from build123d import *

# Parameters (mm, degrees)
EXTRUDE_1_DEPTH = 6
FILLET_1_R      = 3
CHAMFER_1_SIZE  = 3


with BuildPart() as part:
    # 草图1 → 凸台-拉伸1 (new body)
    with BuildSketch(Plane.XY):
        Polygon((-25, 0), (25, 0), (25, 10), (9, 10), (9, 19), (-9, 19), (-9, 10), (-25, 10), align=None)
    extrude(amount=EXTRUDE_1_DEPTH)

    # 圆角1
    fillet_1_edges = [part.edges().sort_by_distance(p)[0] for p in [
        (25, 10, 3),
        (25, 0, 3),
        (-25, 0, 3),
        (-25, 10, 3),
    ]]
    fillet(fillet_1_edges, radius=FILLET_1_R)

    # 倒角1
    chamfer_1_edges = [part.edges().sort_by_distance(p)[0] for p in [
        (0, 19, 6),
        (0, 19, 0),
    ]]
    chamfer(chamfer_1_edges, length=CHAMFER_1_SIZE - 0.0001)  # a hair under: the kernel refuses the full size


solid = part.part
The model under review builds one solid part; all positions refer to its coordinate system, in mm. A direction names the side the tool comes from. Coordinates: 2 decimals unless noted, no trailing zeros. Write each loop counter-clockwise with the first axis right and the second up, starting at its lowest first coordinate (ties: lowest second). Pieces come first, ordered by that corner, then holes. Notation, with made-up numbers: (6, 78) - (26, 78) arc R15 ccw to (26, 95) - close; hole circle Ø7 at (26.25, 23). An arc over 180 degrees is marked (long way). Answer as CSV lines item,"result".
(1) For line 1 along X through (y, z) = (17.5, 2.75); line 2 along Y through (x, z) = (-20, 4); line 3 along X through (y, z) = (2.75, 1), list the stretches that pass through material, from the lowest coordinate up. Write a range as [from, to].
Data:
line 1,"x = [-9, 9]"
line 2,"y = [0, 10]"
line 3,"x = [-24.99, 24.99]"
(2) We need section D-D (x = -21). Give the boundary of the cut face in (y, z), plus the area to 3 significant figures.
Data:
outline,"(0, 0) - (10, 0) - (10, 6) - (0, 6) - close"
area,"60.0 mm2"
(3) Tool access review of faces 1 (the flat face through (16, 10, 3)), 2 (the flat face through (0, 6, 6)), 3 (the flat face through (-15, 10, 3)): name each direction out of +Z, -Z, +X, -X, +Y, -Y from which nothing blocks a thin tool from reaching the whole face with its end or side.
Data:
face 1,"+Z, -Z, +X, +Y"
face 2,"+Z, +X, -X, +Y, -Y"
face 3,"+Z, -Z, -X, +Y"
(4) We need section C-C (y = 13.5). Give the boundary of the cut face in (x, z).
Data:
outline,"(-9, 0) - (9, 0) - (9, 6) - (-9, 6) - close"
(5) We need section B-B (z = 4). Give the boundary of the cut face in (x, y), plus the area to 3 significant figures.
Data:
outline,"(-25, 3) arc R3 ccw to (-22, 0) - (22, 0) arc R3 ccw to (25, 3) - (25, 7) arc R3 ccw to (22, 10) - (9, 10) - (9, 18) - (-9, 18) - (-9, 10) - (-22, 10) arc R3 ccw to (-25, 7) - close"
area,"636 mm2"
(6) Clearance check with flat-ended pins moving along their axes: pin 1 Ø1.5 at (y, z) = (10.5, 1.5) entering from +X; pin 2 Ø3 at (x, z) = (15, 2) entering from +Y; pin 3 Ø1.5 at (y, z) = (9, 3) entering from +X; pin 4 Ø3 at (x, y) = (-13.5, 10.5) entering from -Z. State where each tip first meets the part, or that it passes through.
Data:
pin 1,"stops at x = 23.2"
pin 2,"stops at y = 10"
pin 3,"stops at x = 24.73"
pin 4,"stops at z = 0"
